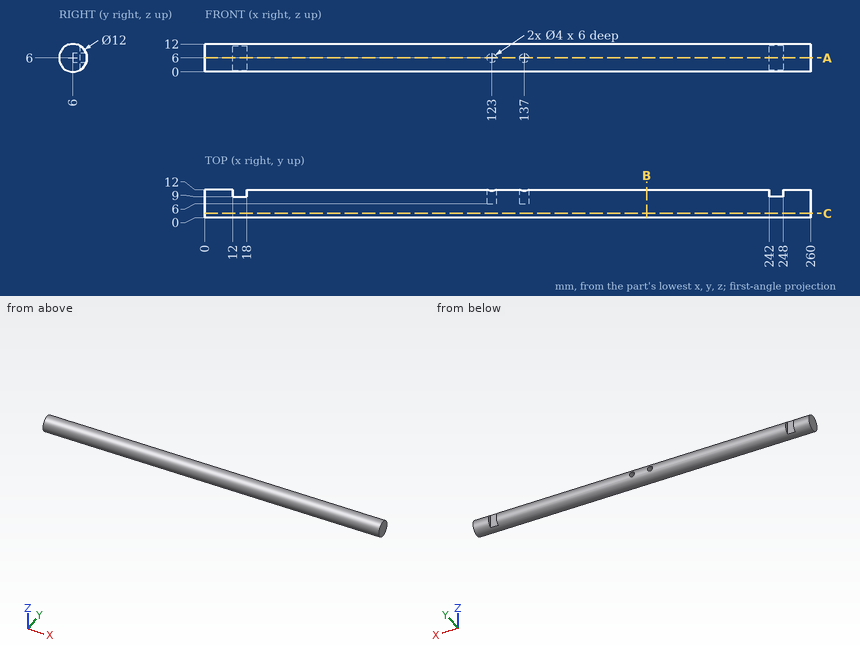
The figure shows three views and two pictorial views of one solid part (mm, origin at its lowest corner). Answer the questions. Coordinates: 2 decimals unless noted, no trailing zeros. Loops run counter-clockwise (first coordinate to the right, second up) from the corner with the lowest first, then second, coordinate; pieces in that order, holes last. Notation, with made-up numbers: (6.5, -35.5) -> (17.5, -35.5) arc R19 ccw to (17.5, -6.5) -> close; hole circle Ø8 at (81, 7.25). An arc over 180 degrees is marked (long way). Return JSON: item names as keys, results as strings. Group by question number.
(1) Find the intervals of material crossed by probe 1 along Y at (x, z) = (88, 5.25); probe 2 along Z at (x, y) = (137, 8.5); probe 3 along Z at (x, y) = (137, 10.5), in increasing order. Write a range as from..to.
(2) Given pin 1 Ø1.5 at (x, z) = (168, 7.5) entering from +Y; pin 2 Ø1.5 at (x, y) = (124.5, 1.5) entering from -Z; pin 3 Ø3 at (x, z) = (16, 4) entering from +Y, each flat-ended and moving along its own axis, determine where each tip first touches the part or whether it passes through.
(3) A cutting plane is placed at C-C on y = 2. Write down the section's boundary in (x, z).
(4) A cutting plane is placed at A-A on z = 6. Write down the section's boundary in (x, y), and give its area (3 significant figures).
(5) A cutting plane is placed at B-B on x = 189.5. Write down the section's boundary in (y, z), and give its area (3 significant figures).
The answers:
{
 "1": {"probe 1": "y = 0.05..11.95", "probe 2": "z = 0.55..4, 8..11.45", "probe 3": "z = 2.03..4, 8..9.97"},
 "2": {"pin 1": "stops at y = 11.95", "pin 2": "stops at z = 1.32", "pin 3": "stops at y = 9"},
 "3": {"outline": "(0, 1.53) -> (260, 1.53) -> (260, 10.47) -> (0, 10.47) -> close"},
 "4": {"outline": "(0, 0) -> (260, 0) -> (260, 12) -> (248, 12) -> (248, 9) -> (242, 9) -> (242, 12) -> (139, 12) -> (139, 6) -> (135, 6) -> (135, 12) -> (125, 12) -> (125, 6) -> (121, 6) -> (121, 12) -> (18, 12) -> (18, 9) -> (12, 9) -> (12, 12) -> (0, 12) -> close", "area": "3,040 mm^2"},
 "5": {"outline": "circle Ø12 at (6, 6)", "area": "113 mm^2"}
}
